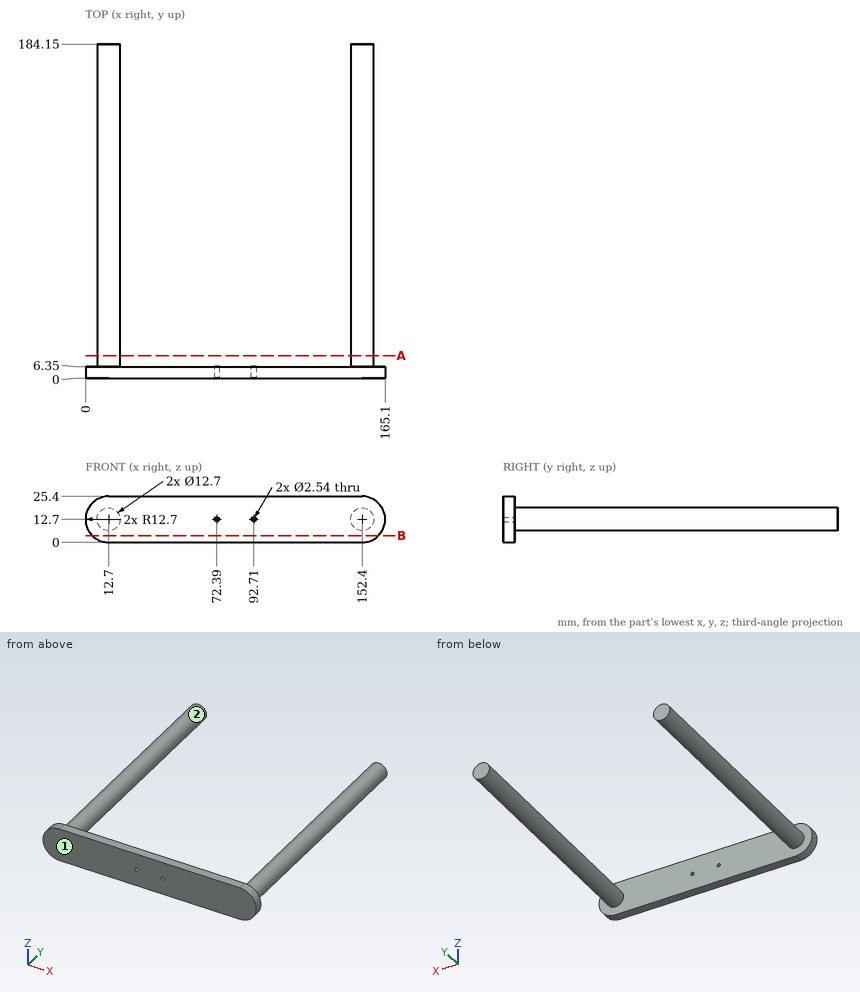
Study the drawing (mm; zero at the part's minimum x, y, z) and answer. A direction names the side the tool comes from. Give positions to 0.01 mm unless a question says otherwise; leave off trailing zeros. Write each loop counter-clockwise with the first axis right and the second up, starting at its lowest first coordinate (ties: lowest second). Pieces come first, ordered by that corner, then holes. Notation, with made-up numbers: (-35, -6.5) -> (8, -6.5) arc R11 ccw to (8, -1.5) -> close; hole circle Ø1 at (8, -7). An arc over 180 degrees is marked (long way). Write item = value, one per line. Start each with the question number.
1) Straight lines are drawn through the part: line 1 along Z through (x, y) = (92.71, 4.25); line 2 along Y through (x, z) = (71, 12.25); line 3 along Z through (x, y) = (72, 2). For each, find the intervals that lie inside material, in ascending order.
2) Which of the six approach directions +Z, -Z, +X, -X, +Y, -Y give full straight-line access (tool end or side, diameter ignored) to the marked faces 1 and 2?
3) The part is cut by section B-B, the plane z = 3.75. Determine the outline of the cut face in (x, y), and give its area (3 significant figures).
4) Each of these flat-tipped pins is pushed along its axis until it touches: pin 1 (2 mm diameter, centred on x = 103.5, z = 5, fed in from -Y); pin 2 (6 mm diameter, centred on y = 111, z = 9, fed in from +X); pin 3 (12.5 mm diameter, centred on x = 45, z = 17.5, fed in from +Y). Where does it stop, or does it pass through?
5) The part is cut by section A-A, the plane y = 12.5. Determine the outline of the cut face in (x, z), and give its area (3 significant figures).
Solutions:
q1.line_1 = 0 to 11.43, 13.97 to 25.4
q1.line_2 = 0 to 6.35
q1.line_3 = 0 to 11.49, 13.91 to 25.4
q2.face_1 = +Z, -Z, +X, -X, -Y
q2.face_2 = +Y
q3.outline = (3.69, 0) -> (161.41, 0) -> (161.41, 6.35) -> (3.69, 6.35) -> close
q3.area = 1,000 mm²
q4.pin_1 = 0
q4.pin_2 = 158.71
q4.pin_3 = 6.35
q5.outline = circle Ø12.7 at (12.7, 12.7); circle Ø12.7 at (152.4, 12.7)
q5.area = 253 mm²
